Geometry: see drawing. Coordinates: mm, zero at the bounding-box minimum. A direction names the side the tool comes from. Round coordinates to 2 decimals unless told otherwise and drop trailing zeros. Loops run counter-clockwise (first coordinate to the right, second up) from the corner with the lowest first, then second, coordinate; pieces in that order, holes last. Notation, with made-up numbers: (60.25, 57) - (67.25, 57) arc R6 ccw to (67.25, 65) - close; hole circle Ø1 at (64, 17.5). An arc over 180 degrees is marked (long way). Write item = value, one per line. Start each with the question number.
Item 1: Section C-C (x = 3). Return loops of the section in (y, z).
Item 2: Line query: line 1 (Y direction, x = 35, z = 1.3); line 2 (X direction, y = 35, z = 2.3); line 3 (X direction, y = 7, z = 4.5). Output: solid intervals per line, ascending. Write a range as from..to.
Item 3: Section A-A (x = 33). Return loops of the section in (y, z), plus the area to 3 significant figures.
Item 4: Section D-D (y = 27.5). Return loops of the section in (x, z), plus the area to 3 significant figures.
Item 5: First-contact query: pin 1 (6 mm diameter, centred on x = 33.5, y = 21, fed in from +Z); pin 2 (1.5 mm diameter, centred on y = 18, z = 1.5, fed in from +X); pin 3 (1 mm diameter, centred on y = 11.5, z = 3.5, fed in from -X); pin 4 (1.8 mm diameter, centred on x = 3, y = 35, fed in from +Z). Flat tips, straight axial feed; report the tip coordinate or a pass-through.
Item 6: Section B-B (z = 2.5). Return loops of the section in (x, y).
Item 7: Access query for the marked faces 5 and 6. Directions: +Z, -Z, +X, -X, +Y, -Y. A direction counts if a zero-diameter tool reaches every point of the face in a straight line with its end or side. Return the directions, or none.
Item 8: Draft query along X for the marked faces 1, 2, 3 and 4. Return one class per face: pulls with the +X half, pulls with the -X half, needs draft (parallel to the pull), parting line crosses it, or undercut.
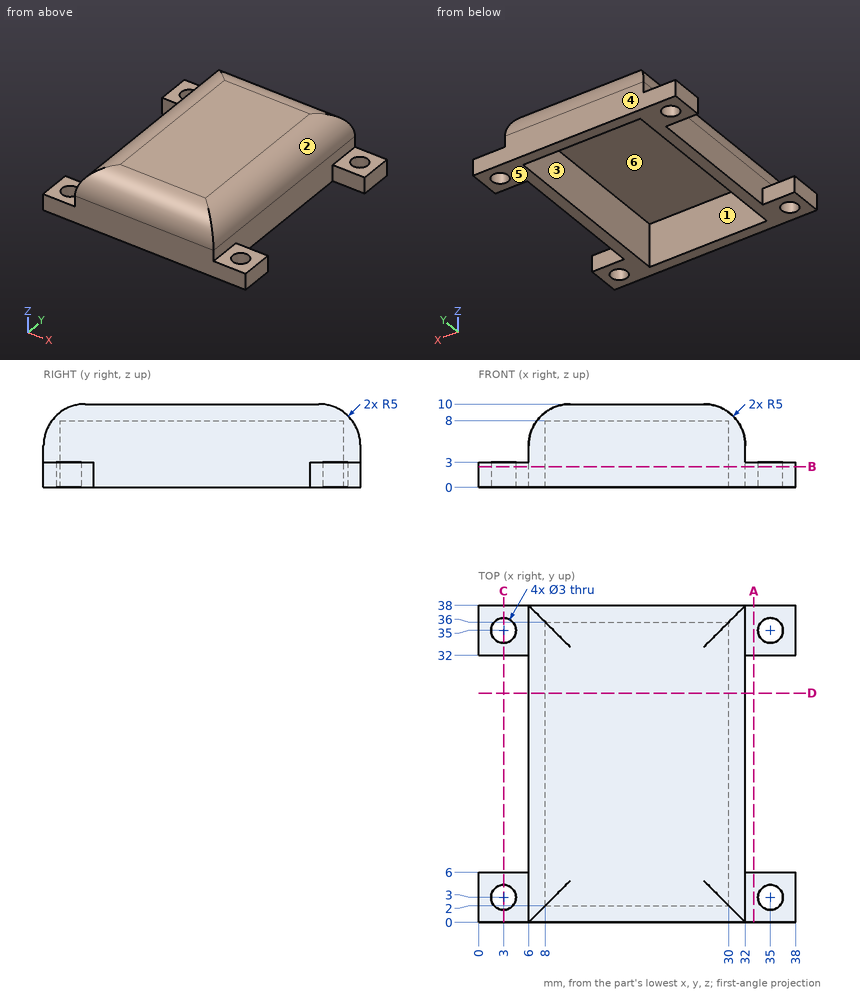
Taken from the geometry:
q1.outline = (0, 0) - (1.5, 0) - (1.5, 3) - (0, 3) - close; (4.5, 0) - (6, 0) - (6, 3) - (4.5, 3) - close; (32, 0) - (33.5, 0) - (33.5, 3) - (32, 3) - close; (36.5, 0) - (38, 0) - (38, 3) - (36.5, 3) - close
q2.line_1 = 0..1.5, 4.5..6, 32..33.5, 36.5..38
q2.line_2 = 0..1.5, 4.5..8, 30..33.5, 36.5..38
q2.line_3 = 6..8, 30..32
q3.outline = (0, 0) - (6, 0) - (6, 3) - (0, 3) - close; (32, 0) - (38, 0) - (38, 3) - (32, 3) - close
q3.area = 36.0 mm^2
q4.outline = (6, 0) - (8, 0) - (8, 8) - (30, 8) - (30, 0) - (32, 0) - (32, 5) arc R5 ccw to (27, 10) - (11, 10) arc R5 ccw to (6, 5) - close
q4.area = 73.3 mm^2
q5.pin_1 = 8.57
q5.pin_2 = 32
q5.pin_3 = 6
q5.pin_4 = through
q6.outline = (0, 0) - (38, 0) - (38, 6) - (32, 6) - (32, 32) - (38, 32) - (38, 38) - (0, 38) - (0, 32) - (6, 32) - (6, 6) - (0, 6) - close; hole circle Ø3 at (3, 3); hole circle Ø3 at (3, 35); hole (8, 2) - (30, 2) - (30, 36) - (8, 36) - close; hole circle Ø3 at (35, 3); hole circle Ø3 at (35, 35)
q7.face_5 = -Z, +X, -X, +Y, -Y
q7.face_6 = -Z
q8.face_1 = undercut
q8.face_2 = pulls with the +X half
q8.face_3 = undercut
q8.face_4 = needs draft
